Read the model definition and answer for the solid it produces. Units are mm, in the model's axes. Give positions to 0.01 mm unless a question says otherwise; leave off trailing zeros. Loops run counter-clockwise (first coordinate to the right, second up) from the corner with the lowest first, then second, coordinate; pieces in that order, holes last.
(1) Find section A-A, the plane x = 184. Write down the section's boundary in (y, z), then the cut area to 3 significant figures.
(2) Determine the mould class of faces 1 (the face through (-36, -160, -1)), 2 (the face through (-118, 118, 0)), 3 (the face through (181.02, 183.14, -1.48)) for opening direction X: pulls with the +X half, pulls with the -X half, needs draft (parallel to the pull), parting line crosses it, or undercut.
(3) Straight lines are drawn through the part: probe 1 along Y at (x, z) = (0, -1.4); probe 2 along X at (y, z) = (135.5, -1.7); probe 3 along Y at (x, z) = (55, -1.25). For each, find the intervals that lie inside material, in ascending order.
(4) Find section D-D, the plane z = -2.4. State how many separate pieces and enclosed holes the cut face has, then the cut area to 3 significant figures.
(5) Each of these flat-tipped pins is pushed along its axis until it touches: P1, Ø11, axis at x = -130.11, y = 130.11, coming from the +Z side; P2, Ø16, axis at x = 0, y = 184, coming from the -Z side. Where does it stop, or does it pass through?
(6) Find section B-B, the plane x = 0. Write down the section's boundary in (y, z).
Autodesk Inventor part; units mm, degrees
ref_plane "YZ Plane" through (0, 0, 0) normal (1, 0, 0) x (0, 1, 0)
ref_plane "XZ Plane" through (0, 0, 0) normal (0, 1, 0) x (-1, 0, 0)
ref_plane "XY Plane" through (0, 0, 0) normal (0, 0, 1) x (1, 0, 0)
sketch "Sketch2" plane through (0, 0, 0) normal (0, 0, 1) x (1, 0, 0)
  line L0 (-257.5, 106.66) -> (-106.66, 257.5)
  line L1 (-106.66, 257.5) -> (106.66, 257.5)
  line L2 (106.66, 257.5) -> (257.5, 106.66)
  line L3 (257.5, 106.66) -> (257.5, -106.66)
  line L4 (257.5, -106.66) -> (106.66, -257.5)
  line L5 (106.66, -257.5) -> (-106.66, -257.5)
  line L6 (-106.66, -257.5) -> (-257.5, -106.66)
  line L7 (-257.5, -106.66) -> (-257.5, 106.66)
  circle A0 centre (0, 0) radius 164
  point P0 (0, 257.5)
  dimension "d23" = 515
  dimension "d26" = 328
extrude "Plate1" add sketch "Sketch2" against normal blind 3
sketch "Sketch4" plane through (0, 0, 0) normal (0, 0, 1) x (1, 0, 0)
  circle A0 centre (0, 184) radius 6.25
  circle A1 centre (0, 0) radius 164
  dimension "d16" = 12.5
  dimension "d17" = 184
extrude "Extrusion1" cut sketch "Sketch4" against normal up to surface (3 mm away) contours A0
pattern_circular "Circular Pattern1" count 8 over 360 about axis through (0, 0, -10) along (0, 0, 1) of "Extrusion1"
equation "\"d23\" = Барабан_размер_по_плоскостям"
equation "\"d15\" = Thickness"
equation "\"BendRadius\" = Thickness"
equation "\"BendReliefWidth\" = Thickness"
equation "\"BendReliefDepth\" = 0.5 * Thickness"
equation "\"CornerReliefSize\" = 4 * Thickness"
equation "\"MinimumRemnant\" = 2 * Thickness"
equation "\"TransitionRadius\" = BendRadius"
equation "\"JacobiRadiusSize\" = BendRadius"
equation "\"GapSize\" = Thickness"
properties part number "DMF 01 22 Барабан торец КОРМА v2.1"
Entries:
1. outline: (-180.16, -3) - (-6.25, -3) - (-6.25, 0) - (-180.16, 0) - close; (6.25, -3) - (180.16, -3) - (180.16, 0) - (6.25, 0) - close
1. area: 1,040 mm2
2. face 1: undercut
2. face 2: needs draft
2. face 3: pulls with the +X half
3. probe 1: y = -257.5 to -190.25, -177.75 to -164, 164 to 177.75, 190.25 to 257.5
3. probe 2: x = -228.66 to -133.27, -126.95 to -92.39, 92.39 to 126.95, 133.27 to 228.66
3. probe 3: y = -257.5 to -154.5, 154.5 to 257.5
4. separate pieces: 1
4. enclosed holes: 9
4. area: 134,000 mm2
5. P1: passes through
5. P2: stops at z = -3
6. outline: (-257.5, -3) - (-190.25, -3) - (-190.25, 0) - (-257.5, 0) - close; (-177.75, -3) - (-164, -3) - (-164, 0) - (-177.75, 0) - close; (164, -3) - (177.75, -3) - (177.75, 0) - (164, 0) - close; (190.25, -3) - (257.5, -3) - (257.5, 0) - (190.25, 0) - close
